Autodesk Inventor part; units mm, degrees
ref_plane "YZ Plane" through (0, 0, 0) normal (1, 0, 0) x (0, 1, 0)
ref_plane "XZ Plane" through (0, 0, 0) normal (0, 1, 0) x (-1, 0, 0)
ref_plane "XY Plane" through (0, 0, 0) normal (0, 0, 1) x (1, 0, 0)
sketch "Sketch1" plane through (0, 0, 0) normal (0, 0, 1) x (1, 0, 0)
  circle A0 centre (0, 0) radius 6.35
  dimension "d0" = 12.7
extrude "Internal 1/2\" Round" add sketch "Sketch1" against normal blind 7.9375
sketch "Sketch2" plane through (0, 0, -7.9375) normal (0, 0, -1) x (-1, 0, 0)
  circle A0 centre (0, 0) radius 6.35
  line L0 (3.6662, 6.35) -> (7.3323, 0)
  line L1 (7.3323, 0) -> (3.6662, -6.35)
  line L2 (3.6662, -6.35) -> (-3.6662, -6.35)
  line L3 (-3.6662, -6.35) -> (-7.3323, 0)
  line L4 (-7.3323, 0) -> (-3.6662, 6.35)
  line L5 (-3.6662, 6.35) -> (3.6662, 6.35)
extrude "Pulley 1/2\" Hex" add sketch "Sketch2" along normal blind 38.1
sketch "Sketch3" plane through (0, 0, -46.0375) normal (0, 0, -1) x (-1, 0, 0)
  circle A0 centre (0, 0) radius 6.35
extrude "External 1/2\" Round" add sketch "Sketch3" along normal blind 7.9375
sketch "Sketch4" plane through (0, 0, -53.975) normal (0, 0, -1) x (-1, 0, 0)
  circle A0 centre (0, 0) radius 6.35
  line L0 (3.2748, 5.4404) -> (6.3489, 0.1158)
  line L1 (6.3489, -0.1158) -> (3.2748, -5.4404)
  line L2 (3.0742, -5.5563) -> (-3.0742, -5.5563)
  line L3 (-3.2748, -5.4404) -> (-6.3489, -0.1158)
  line L4 (-6.3489, 0.1158) -> (-3.2748, 5.4404)
  line L5 (-3.0742, 5.5562) -> (3.0742, 5.5562)
  dimension "d7" = 11.1125
extrude "Wheel 7/16\" Hex" add sketch "Sketch4" along normal blind 44.45 contours A0 L1 L2 L3 L4 L5 L0
sketch "Sketch6" plane through (0, 0, -98.425) normal (0, 0, -1) x (-1, 0, 0)
  arc A0 (6.3489, -0.1158) -> (6.3489, 0.1158) centre (0, 0) ccw
sketch "Sketch5" plane through (0, 0, 0) normal (0, 0, 1) x (1, 0, 0)
  circle A0 centre (0, 0) radius 6.35
hole "Internal 1/4\"-20 Tap" at (0, 0, 0) direction (0, 0, -1) diameter 4.9784 depth 19.05 tip angle 118
hole "External 1/4\"-20 Tap" at (0, 0, -98.425) direction (0, 0, 1) diameter 4.9784 depth 19.05 tip angle 118
properties part number "Live Axle" material "Aluminum 7075"
Verification items for the finished model (mm, model axes). A direction names the side the tool comes from. Give positions to 0.01 mm unless a question says otherwise; leave off trailing zeros. Loops run counter-clockwise (first coordinate to the right, second up) from the corner with the lowest first, then second, coordinate; pieces in that order, holes last. Notation, with made-up numbers: (-18, -14.75) - (-5, -14.75) arc R22 ccw to (-5, 12.25) - close; hole circle Ø1 at (-4, -5.75). An arc over 180 degrees is marked (long way). Write item = value, one per line. Start each with the question number.
Q1. Cross-section at D-D, the plane z = -84.5. Enter the section's corners in (x, y).
Q2. Mould release check, pull along X, two halves, no side actions. Record for faces 1 (the face through (-0.422, -0.094, -78.139)), 2 (the face through (5.474, -3.219, -26.721)), 3 (the face through (-5, -3, -53.975)): released by +X, released by -X, zero draft, split by the parting line, or undercut.
Q3. Tool access check on faces 4 (the face through (-3, -6, -7.938)), 5 (the face through (4.833, 2.741, -75.889)), 6 (the face through (0, 5.556, -76)), 7 (the face through (-7, 0, -46.038)), 8 (the face through (4.8, -2.8, -75.9)). Record the directions out of +Z, -Z, +X, -X, +Y, -Y that give a thin tool (end or side, any length) a straight path to the whole face; none if there is none.
Q4. Cross-section at C-C, the plane z = -59.5. Enter the section's corners in (x, y).
Q5. Depth check by flat-ended pin: P1, Ø1.5, axis at y = 2.5, z = -75.5, coming from the +X side; P2, Ø0.6, axis at x = 1.5, y = -6, coming from the -Z side (3 decimals); P3, Ø2, axis at x = 0.5, z = -73.5, coming from the +Y side. Enter the tip coordinate at first touch or a pass-through.
Q6. Thickness scan on line 1 (X direction, y = 0, z = -6.25); line 2 (X direction, y = 0, z = -15). Record the ranges inside material, lowest first.
Q7. Cross-section at A-A, the plane z = -18. Enter the section's corners in (x, y), and give its area (3 significant figures).
Answer key:
q1.outline = (-6.35, -0.12) - (-3.27, -5.44) arc R6.35 ccw to (-3.07, -5.56) - (3.07, -5.56) arc R6.35 ccw to (3.27, -5.44) - (6.35, -0.12) arc R6.35 ccw to (6.35, 0.12) - (3.27, 5.44) arc R6.35 ccw to (3.07, 5.56) - (-3.07, 5.56) arc R6.35 ccw to (-3.27, 5.44) - (-6.35, 0.12) arc R6.35 ccw to start; hole circle Ø4.98 at (0, 0)
q2.face_1 = undercut
q2.face_2 = released by +X
q2.face_3 = zero draft
q3.face_4 = +Z, -X, -Y
q3.face_5 = -Z, +X, +Y
q3.face_6 = -Z, +X, -X, +Y
q3.face_7 = -Z, -X
q3.face_8 = -Z, +X, -Y
q4.outline = (-6.35, -0.12) - (-3.27, -5.44) arc R6.35 ccw to (-3.07, -5.56) - (3.07, -5.56) arc R6.35 ccw to (3.27, -5.44) - (6.35, -0.12) arc R6.35 ccw to (6.35, 0.12) - (3.27, 5.44) arc R6.35 ccw to (3.07, 5.56) - (-3.07, 5.56) arc R6.35 ccw to (-3.27, 5.44) - (-6.35, 0.12) arc R6.35 ccw to start
q5.P1 = 5.41
q5.P2 = -53.975
q5.P3 = 5.56
q6.line_1 = -6.35 to -2.49, 2.49 to 6.35
q6.line_2 = -7.33 to -2.49, 2.49 to 7.33
q7.outline = (-7.33, 0) - (-3.67, -6.35) - (3.67, -6.35) - (7.33, 0) - (3.67, 6.35) - (-3.67, 6.35) - close; hole circle Ø4.98 at (0, 0)
q7.area = 120 mm^2
